Design review of the part shown in the three views and the two pictorial views. Dimensions are in mm from the part's minimum x, y and z. A direction names the side the tool comes from. Round coordinates to 2 decimals unless told otherwise and drop trailing zeros. Order: outer loops, then holes, each group sorted by start corner. A loop starts at its lowest first (then second) coordinate and runs counter-clockwise, first axis right, second up.
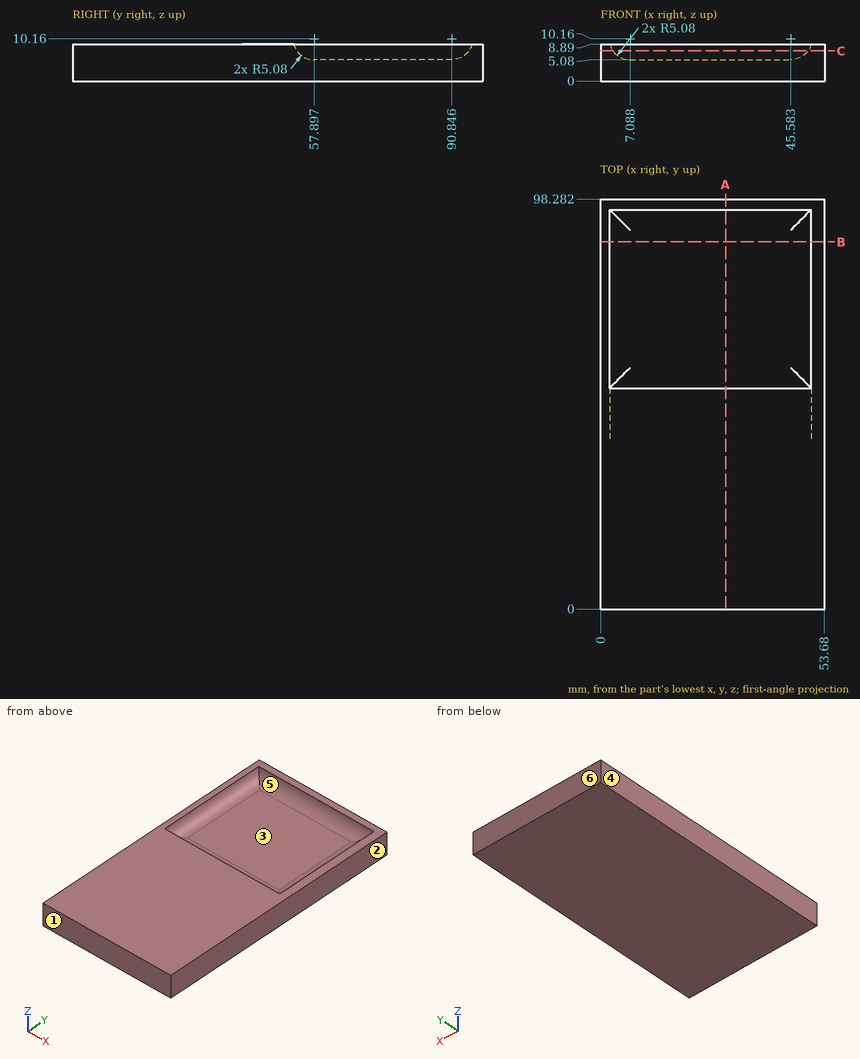
1) The part is to be moulded in two halves that separate along X. For the marked faces 1, 2, 3 and 4, say which applies: released by +X, released by -X, zero draft, split by the parting line, or undercut.
Results:
face 1: zero draft
face 2: released by +X
face 3: undercut
face 4: released by -X
2) Clearance check with flat-ended pins moving along their axes: P1, Ø16.5, axis at x = 19, y = 78.5, coming from the +Z side; P2, Ø5, axis at x = 44.5, y = 55, coming from the -Z side. State where each tip first meets the part, or that it passes through.
Results:
P1: stops at z = 5.08
P2: stops at z = 0
3) Take a section at C-C on z = 7.25. Give the boundary of the cut face in (x, y) (1 decimal).
Results:
outline: (0, 0) - (53.7, 0) - (53.7, 98.3) - (0, 98.3) - close; hole (2.9, 53.7) - (49.7, 53.7) - (49.7, 95) - (2.9, 95) - close
4) Take a section at B-B on y = 88. Give the boundary of the cut face in (x, z).
Results:
outline: (0, 0) - (53.68, 0) - (53.68, 8.89) - (50.5, 8.89) arc R5.08 cw to (45.58, 5.08) - (7.09, 5.08) arc R5.08 cw to (2.17, 8.89) - (0, 8.89) - close
5) Take a section at A-A on x = 30. Give the boundary of the cut face in (y, z) (1 decimal).
Results:
outline: (0, 0) - (98.3, 0) - (98.3, 8.9) - (95.8, 8.9) arc R5.1 cw to (90.8, 5.1) - (57.9, 5.1) arc R5.1 cw to (53, 8.9) - (0, 8.9) - close
6) To check wall thickness, follow line 1 along Z through (x, y) = (10.5, 61); line 2 along Y through (x, z) = (26.5, 6.25) (1 decimal); line 3 along Y through (x, z) = (18, 6.5) (1 decimal). State the ranges of each line that lie inside material, in increasing order.
Results:
line 1: z = 0 to 5.08
line 2: y = 0 to 54.7, 94.1 to 98.3
line 3: y = 0 to 54.4, 94.4 to 98.3
7) For the marked faces 5 and 6, list the 3-axis set-ups (+Z, -Z, +X, -X, +Y, -Y) from which the entire face can be reached by the end or side of a thin tool; tool diameter is ignored.
Results:
face 5: +Z
face 6: +Z, -Z, +X, -X, +Y
